Source: CAD feature listing. Evaluate the final solid. Frame: model axes, mm. A direction names the side the tool comes from. Coordinates: 2 decimals unless noted, no trailing zeros. Write each loop counter-clockwise with the first axis right and the second up, starting at its lowest first coordinate (ties: lowest second). Pieces come first, ordered by that corner, then holes. Notation, with made-up numbers: (-14.5, 82) -> (7.5, 82) arc R23 ccw to (7.5, 116) -> close; hole circle Ø10 at (4.25, 88.25). An arc over 180 degrees is marked (long way). Write item = value, one per line.
from build123d import *

# Parameters (mm, degrees)
CHAMFER1_SIZE = 0.2


with BuildPart() as part:
    # Sketch1 → Revolve1 (revolve)
    with BuildSketch(Plane.XY, mode=Mode.PRIVATE) as revolve1_sk:
        Polygon((0.95, -9.336734694), (0.95, -7.336734694), (4.875, 48.663265306), (4.875, 60.663265306), (6.5, 60.663265306), (6.5, 63.663265306), (4.15, 63.663265306), (4.15, 67.663265306), (2.648417251, 69.46850915), (4.15, 69.46850915), (2.648417251, 71.273752994), (4.15, 71.273752994), (2.648417251, 73.078996837), (4.15, 73.078996837), (2.648417251, 74.884240681), (4.15, 74.884240681), (2.648417251, 76.689484525), (4.15, 76.689484525), (1.474206394, 84.510756718), (1, 84.510756718), (1, 68.96850915), (2, 63.663265306), (2, 60.663265306), (0.275, -7.002676295), (0.275, -8.336734694), (0.575, -8.336734694), (0.575, -9.336734694), align=None)
    revolve(revolve1_sk.sketch.rotate(Axis((0, 103.014460247, 0), (0, -1, 0)), 90), axis=Axis((0, 103.014460247, 0), (0, -1, 0)))

    # Chamfer1
    chamfer1_edges = [part.edges().sort_by_distance(p)[0] for p in [
        (0, -9.336734694, -0.575),
    ]]
    chamfer(chamfer1_edges, length=CHAMFER1_SIZE)


solid = part.part
1) Cut plane B-B, the plane z = -3.25. Give the number of separate pieces and of enclosed holes in the cut face, and give its area (3 significant figures).
Answer block:
separate_pieces = 6
enclosed_holes = 0
area = 276 mm2
2) First-contact query: pin 1 Ø4 at (y, z) = (43, 2) entering from +X; pin 2 Ø6.5 at (x, z) = (1.5, 2) entering from -Y; pin 3 Ø0.7 at (x, z) = (0, 0) entering from -Y; pin 4 Ø1.5 at (y, z) = (9.5, 4) entering from +X. Flat tips, straight axial feed; report the tip coordinate or a pass-through.
Answer block:
pin_1 = 4.54
pin_2 = -9.34
pin_3 = -8.34
pin_4 = through
3) Material intervals for probe 1 along X at (y, z) = (-8.7, 0) (3 decimals); probe 2 along Y at (x, z) = (5.25, -3); probe 3 along Z at (x, y) = (-0.5, 11), sorted ascending. Write a range as [from, to].
Answer block:
probe_1 = [-0.95, -0.575], [0.575, 0.95]
probe_2 = [60.66, 63.66]
probe_3 = [-2.18, -0.54], [0.54, 2.18]
4) Reachability of faces 1 (the cylindrical face through (1, 77, 0)), 2 (the flat face through (-5, 60.663, -1)), 3 (the flat face through (3, 76.689, 0)) from +Z, -Z, +X, -X, +Y, -Y: full face, straight path, thin tool, end or side. Return the list, or none.
Answer block:
face_1 = +Y
face_2 = -Y
face_3 = none
5) Cut plane C-C, the plane y = 66.5. Output: boundary loops of the cut face in (x, z).
Answer block:
outline = circle Ø8.3 at (0, 0); hole circle Ø2.93 at (0, 0)
6) Pull-direction query (Y, two-part tool) for faces 4 (the conical face through (-0.129, 21.055, -2.937)), 5 (the flat face through (3, 73.079, 0)), 6 (the cylindrical face through (3.955, 62.184, -5.158)); classes: +Y half, -Y half, draft (parallel to the pull), parting line (faces both ways), or undercut.
Answer block:
face_4 = -Y half
face_5 = undercut
face_6 = draft
7) Cut plane A-A, the plane y = 38. Output: boundary loops of the cut face in (x, z), and give its area (3 significant figures).
Answer block:
outline = circle Ø8.26 at (0, 0); hole circle Ø2.84 at (0, 0)
area = 47.2 mm2
